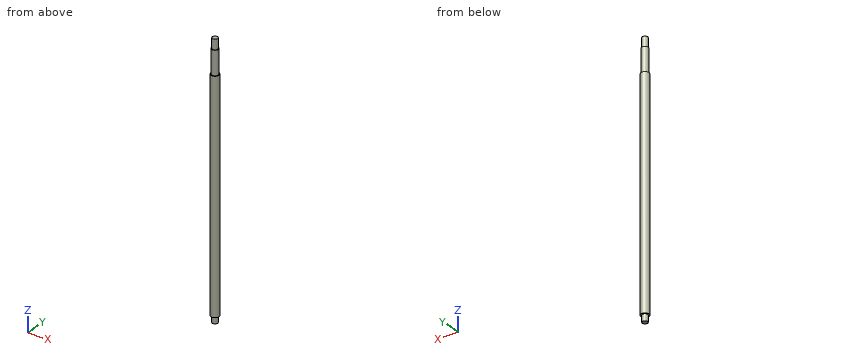
from build123d import *

# Parameters (mm, degrees)
SKETCH_1_R          = 6
EXTRUDE_1_DEPTH     = 400
SKETCH_2_OUTSIDE_W  = 94.072
SKETCH_2_OUTSIDE_H  = 94.072
SKETCH_2_OUTSIDE_R  = 5
CUT_EXTRUDE_1_DEPTH = 51
SKETCH_4_OUTSIDE_W  = 94.072
SKETCH_4_OUTSIDE_H  = 94.072
SKETCH_4_OUTSIDE_R  = 4
CUT_EXTRUDE_3_DEPTH = 15
SKETCH_5_OUTSIDE_W  = 94.072
SKETCH_5_OUTSIDE_H  = 94.072
SKETCH_5_OUTSIDE_R  = 4
CUT_EXTRUDE_4_DEPTH = 10


with BuildPart() as part:
    # Эскиз1 → Бобышка-Вытянуть1 (new body)
    with BuildSketch(Plane.XY):
        Circle(SKETCH_1_R)
    extrude(amount=EXTRUDE_1_DEPTH)

    # Эскиз2 outside → Вырез-Вытянуть1 (cut)
    with BuildSketch(Plane.XY.offset(400)):
        Rectangle(SKETCH_2_OUTSIDE_W, SKETCH_2_OUTSIDE_H)
        Circle(SKETCH_2_OUTSIDE_R, mode=Mode.SUBTRACT)
    extrude(amount=-CUT_EXTRUDE_1_DEPTH, mode=Mode.SUBTRACT)

    # Эскиз4 outside → Вырез-Вытянуть3 (cut)
    with BuildSketch(Plane.XY.offset(400)):
        Rectangle(SKETCH_4_OUTSIDE_W, SKETCH_4_OUTSIDE_H)
        Circle(SKETCH_4_OUTSIDE_R, mode=Mode.SUBTRACT)
    extrude(amount=-CUT_EXTRUDE_3_DEPTH, mode=Mode.SUBTRACT)

    # Эскиз5 outside → Вырез-Вытянуть4 (cut)
    with BuildSketch(Plane(origin=(0, 0, 0), x_dir=(-1, 0, 0), z_dir=(0, 0, -1))):
        Rectangle(SKETCH_5_OUTSIDE_W, SKETCH_5_OUTSIDE_H)
        with Locations(Location((0, 0, 0), (0, 0, 180))):
            Circle(SKETCH_5_OUTSIDE_R, mode=Mode.SUBTRACT)
    extrude(amount=-CUT_EXTRUDE_4_DEPTH, mode=Mode.SUBTRACT)


solid = part.part
The model under review builds one solid part; all positions refer to its coordinate system, in mm. Give positions to 0.01 mm unless a question says otherwise; leave off trailing zeros. Order: outer loops, then holes, each group sorted by start corner. A loop starts at its lowest first (then second) coordinate and runs counter-clockwise, first axis right, second up. Notation, with made-up numbers: M -35.75,64.25 L 21.25,64.25 A10 cw 21.25,72.25 Z; hole C 2.25,32 d9. An arc over 180 degrees is marked long. Answer in a Markdown table with one row per item. Add a question column.
1. To check wall thickness, follow line 1 along Y through (x, z) = (0.5, 22); line 2 along Y through (x, z) = (-4.5, 302); line 3 along X through (y, z) = (-0.25, 63). State the ranges of each line that lie inside material, in increasing order.
2. For pin 1 Ø1.5 at (x, z) = (-4.5, 223.5) entering from -Y; pin 2 Ø2 at (x, z) = (1.5, 105) entering from +Y; pin 3 Ø4 at (x, z) = (-2, 150.5) entering from -Y; pin 4 Ø3 at (y, z) = (4.5, 90.5) entering from -X, all flat-tipped, find the tip position at first contact; note any pin that passes through.
3. Add section A-A on x = 0. State the section outline as (y, z) points.
4. Add section C-C on z = 35. State the section outline as (x, y) points, plus the area to 3 significant figures.
The answers:
| question | item | result |
|---|---|---|
| 1 | line 1 | -5.98 to 5.98 |
| 1 | line 2 | -3.97 to 3.97 |
| 1 | line 3 | -5.99 to 5.99 |
| 2 | pin 1 | y = -4.68 |
| 2 | pin 2 | y = 5.98 |
| 2 | pin 3 | y = -6 |
| 2 | pin 4 | x = -5.2 |
| 3 | outline | M -6,10 L -4,10 L -4,0 L 4,0 L 4,10 L 6,10 L 6,349 L 5,349 L 5,385 L 4,385 L 4,400 L -4,400 L -4,385 L -5,385 L -5,349 L -6,349 Z |
| 4 | outline | C 0,0 d12 |
| 4 | area | 113 mm2 |
